from build123d import *

# Parameters (mm, degrees)
F1_DEPTH = 63.5
F2_DEPTH = 7.9375
F3_R     = 6.35
F0_W     = 25.4
F0_H     = 19.05
F4_DEPTH = 25.4


with BuildPart() as f1:
    # F0 (on Front) → F1 (new body, symmetric)
    with BuildSketch(Plane.XZ):
        Polygon((22.225, 9.525), (-41.275, 9.525), (-41.275, -9.525), (41.275, -9.525), (41.275, 9.525), align=None)
    extrude(amount=F1_DEPTH, both=True)

    # F0 (on Front) → F2 (join, symmetric)
    with BuildSketch(Plane.XZ):
        with BuildLine():
            add(Edge.make_bspline(
                [(-41.275, 9.525), (-41.2262459326, 39.0642297135), (9.9785681568, 60.561025247), (55.4924441738, 61.8858436616)],
                knots=[0, 0, 0, 0, 110.1650615003, 110.1650615003, 110.1650615003, 110.1650615003], degree=3))
            Line((-41.275, 9.525), (22.225, 9.525))
            Line((22.225, 9.525), (22.225, 27.0002))
            ThreePointArc((22.225, 27.0002), (31.8750542807, 51.1027464191), (55.4924441738, 61.8858436616))
        make_face()
    extrude(amount=F2_DEPTH, both=True)

    # F3
    f3_edges = [f1.edges().sort_by_distance(p)[0] for p in [
        (-41.275, -63.5, 0),
        (41.275, -63.5, 0),
        (41.275, 63.5, 0),
        (-41.275, 63.5, 0),
    ]]
    fillet(f3_edges, radius=F3_R)

    # F0 (on Front) → F4 (join, symmetric)
    with BuildSketch(Plane.XZ):
        with BuildLine():
            Line((22.225, 27.0002), (22.225, 9.525))
            Line((22.225, 9.525), (41.275, 9.525))
            Line((41.275, 9.525), (41.275, 27.0002))
            ThreePointArc((41.275, 27.0002), (45.9246798487, 38.2255201513), (57.15, 42.8752))
            Line((57.15, 42.8752), (59.2859117566, 42.8752))
            Line((59.2859117566, 42.8752), (59.2859117566, 61.9252))
            Line((59.2859117566, 61.9252), (57.15, 61.9252))
            add(Edge.make_bspline(
                [(55.4924441738, 61.8858436616), (56.0458381711, 61.9019518603), (56.5983908409, 61.9150779074), (57.15, 61.9252)],
                knots=[110.1650615003, 110.1650615003, 110.1650615003, 110.1650615003, 111.5045361635, 111.5045361635, 111.5045361635, 111.5045361635], degree=3))
            ThreePointArc((55.4924441738, 61.8858436616), (31.8750542807, 51.1027464191), (22.225, 27.0002))
        make_face()
        with Locations((71.9859117566, 52.4002)):
            Rectangle(F0_W, F0_H)
    extrude(amount=F4_DEPTH, both=True)

    # F0 (on Front) → F5 (revolve)
    with BuildSketch(Plane.XZ):
        Polygon((84.6859117566, 66.675), (84.6859117566, 61.9252), (84.6859117566, 42.8752), (84.6859117566, 38.1), (110.0859117566, 38.1), (110.0859117566, 66.675), align=None)
    revolve(axis=Axis((84.6859117566, 0, 52.3875), (0, 0, 1)))


solid = f1.part
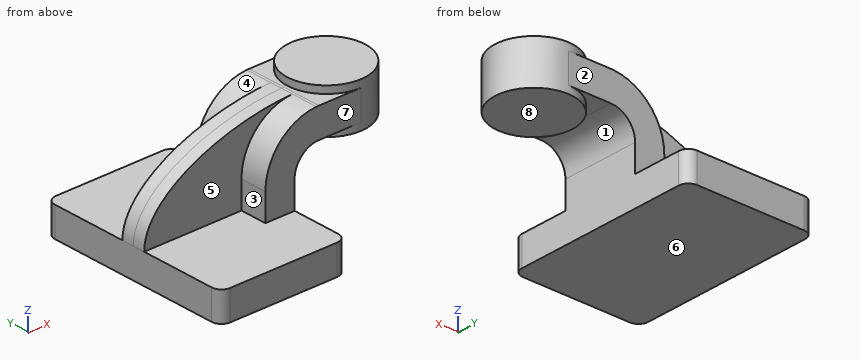
Input: part model. Units: mm. Frame: model coordinates. Face numbers are marked on the shaded views. A direction names the side the tool comes from. Give positions to 0.01 mm unless a question says otherwise; leave off trailing zeros. Loops run counter-clockwise (first coordinate to the right, second up) from the corner with the lowest first, then second, coordinate; pieces in that order, holes last. Notation, with made-up numbers: (-21, 27) - (33, 27) arc R36 cw to (33, 64) - close; hole circle Ø6 at (-32.5, 5.25). An arc over 180 degrees is marked (long way). Use CSV: the item, a comma, the result in double quotes. Start each with the question number.
Item 1: Section B-B on x = 98. Return loops of the section in (y, z) (3 decimals).
Item 2: Reachability of the marked faces 4, 5, 6, 7 and 8 from +Z, -Z, +X, -X, +Y, -Y: full face, straight path, thin tool, end or side. Return the list, or none.
Item 3: Contact query for flat-ended pins moving along their axis: P1, Ø15, axis at x = 96, y = 4, coming from the -Z side; P2, Ø16.5, axis at x = -14.5, y = -29, coming from the +Z side (3 decimals); P3, Ø10, axis at y = -19, z = 4.5, coming from the +X side (3 decimals); P4, Ø3, axis at x = 43, y = -29, coming from the -Z side. Output: stop coordinate, or through.
Item 4: Line query: line 1 (X direction, y = -21.5, z = 11) (3 decimals); line 2 (Y direction, x = -24, z = 31); line 3 (Z direction, x = 56.5, y = 8). Output: solid intervals per line, ascending.
Item 5: Section A-A on y = 40. Return loops of the section in (x, z) (3 decimals), then the cut area to 3 significant figures.
Item 6: Mould query, pull axis X, two halves, no side actions, for the marked faces 1, 2 and 3. Classes: pulls with the +X half, pulls with the -X half, needs draft (parallel to the pull), parting line crosses it, or undercut.
Ans:
1,outline,"(-21.631, 38.1) - (21.631, 38.1) - (21.631, 66.675) - (-21.631, 66.675) - close"
2,face 4,"+Z, -X, +Y"
2,face 5,"+Z, -X, -Y"
2,face 6,"-Z, +X, -X, +Y, -Y"
2,face 7,"+Z, +X, -X, -Y"
2,face 8,"-Z, +X, +Y, -Y"
3,P1,"stops at z = 38.1"
3,P2,"stops at z = 9.525"
3,P3,"stops at x = 41.275"
3,P4,"passes through"
4,line 1,"x = 22.225 to 41.275"
4,line 2,"y = -7.94 to 7.94"
4,line 3,"z = 42.86 to 61.91"
5,outline,"(-41.275, -9.525) - (41.275, -9.525) - (41.275, 9.525) - (-41.275, 9.525) - close"
5,area,"1,570 mm2"
6,face 1,"undercut"
6,face 2,"needs draft"
6,face 3,"pulls with the -X half"
